Print and shaded views of the part. All mm, measured from the part's lowest x, y and z. A direction names the side the tool comes from. Round coordinates to 2 decimals unless told otherwise and drop trailing zeros. Order: outer loops, then holes, each group sorted by start corner. A loop starts at its lowest first (then second) coordinate and runs counter-clockwise, first axis right, second up. Notation, with made-up numbers: (32.25, 72) - (41.25, 72) arc R15 cw to (41.25, 83) - close; hole circle Ø11 at (9.5, -20.75). An arc over 180 degrees is marked (long way). Return JSON: item names as keys, results as strings. Group by question number.
Item 1: Saw through at B-B on x = 24.9. List the corners of the cut face in (y, z), and give its area (3 significant figures).
Item 2: Saw through at C-C on z = 1. List the corners of the cut face in (x, y) (1 decimal).
Item 3: Saw through at D-D on y = 41. List the corners of the cut face in (x, z).
Item 4: Two-plate mould, pull along Y, no slides. Class the marked faces 5, 6 and 7: released by +Y, released by -Y, zero draft, split by the parting line, or undercut.
Item 5: Drop flat-ended pins along their axis: pin 1 (1.8 mm diameter, centred on x = 1.5, z = 2, fed in from +Y); pin 2 (3 mm diameter, centred on y = 48, z = 2.5, fed in from -X); pin 3 (4 mm diameter, centred on y = 2.5, z = 2.5, fed in from +X) (1 decimal); pin 4 (4 mm diameter, centred on y = 20.5, z = 8.5, fed in from -X). Give the stop position or say it passes through.
Item 6: Tool access for the marked faces 1, 2, 3 and 4: list every direction of +Z, -Z, +X, -X, +Y, -Y with a clear straight run to the whole face (end or side of a thin tool).
Item 7: Probe probe 1 along Y at (x, z) = (33, 2.25); probe 2 along X at (y, z) = (36, 4.5); probe 3 along Z at (x, y) = (9, 5.5). List the from-to ranges inside material, lowest first.
Item 8: Saw through at A-A on y = 16.5. List the corners of the cut face in (x, z).
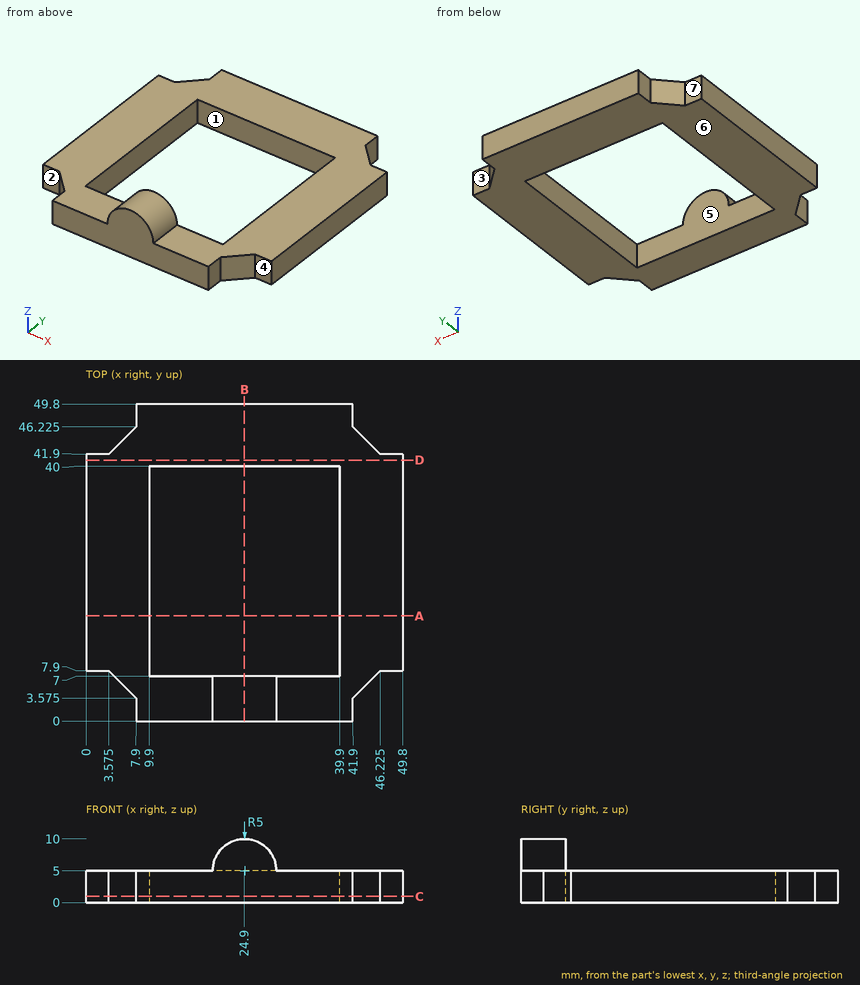
Filled in:
{
 "1": {"outline": "(0, 0) - (7, 0) - (7, 10) - (0, 10) - close; (40, 0) - (49.8, 0) - (49.8, 5) - (40, 5) - close", "area": "119 mm^2"},
 "2": {"outline": "(0, 7.9) - (3.6, 7.9) - (7.9, 3.6) - (7.9, 0) - (41.9, 0) - (41.9, 3.6) - (46.2, 7.9) - (49.8, 7.9) - (49.8, 41.9) - (46.2, 41.9) - (41.9, 46.2) - (41.9, 49.8) - (7.9, 49.8) - (7.9, 46.2) - (3.6, 41.9) - (0, 41.9) - close; hole (9.9, 7) - (39.9, 7) - (39.9, 40) - (9.9, 40) - close"},
 "3": {"outline": "(0, 0) - (49.8, 0) - (49.8, 5) - (0, 5) - close"},
 "4": {"face 5": "undercut", "face 6": "zero draft", "face 7": "released by +Y"},
 "5": {"pin 1": "stops at y = 41.9", "pin 2": "stops at x = 7.9", "pin 3": "stops at x = 42.8", "pin 4": "passes through"},
 "6": {"face 1": "+Z, -Z", "face 2": "+Z, -Z, -X, -Y", "face 3": "+Z, -Z, +X, +Y", "face 4": "+Z, -Z, +X, -Y"},
 "7": {"probe 1": "y = 0 to 7, 40 to 49.8", "probe 2": "x = 0 to 9.9, 39.9 to 49.8", "probe 3": "z = 0 to 5"},
 "8": {"outline": "(0, 0) - (9.9, 0) - (9.9, 5) - (0, 5) - close; (39.9, 0) - (49.8, 0) - (49.8, 5) - (39.9, 5) - close"}
}
